```python
from build123d import *

# Parameters (mm, degrees)
BOX001_W          = 30
BOX001_H          = 70
BOX001_DEPTH      = 7.5
CYLINDER003_R     = 5
CYLINDER003_DEPTH = 40
CYLINDER002_R     = 17.5
CYLINDER002_DEPTH = 20


with BuildPart() as cube001:
    # Box001 → Box001 (new body)
    with BuildSketch(Plane(origin=(7, -20, 9), x_dir=(1, 0, 0), z_dir=(0, 0, 1))):
        with Locations((15, 35)):
            Rectangle(BOX001_W, BOX001_H)
    extrude(amount=BOX001_DEPTH)


with BuildPart() as cylinder003:
    # Cylinder003 → Cylinder003 (new body)
    with BuildSketch(Plane.XY.offset(-10)):
        Circle(CYLINDER003_R)
    extrude(amount=CYLINDER003_DEPTH)


with BuildPart() as mount_top:
    # Cylinder002 → Cylinder002 (new body)
    with BuildSketch(Plane.XY):
        Circle(CYLINDER002_R)
    extrude(amount=CYLINDER002_DEPTH)

    # Cut002: cut Cylinder003
    add(cylinder003.part, mode=Mode.SUBTRACT)

    # Cut003: cut Cube001
    add(cube001.part, mode=Mode.SUBTRACT)


solid = mount_top.part
```
Here's how the part is built. I have some questions about the finished solid (model axes, mm). A direction names the side the tool comes from. Coordinates: 2 decimals unless noted, no trailing zeros. Write each loop counter-clockwise with the first axis right and the second up, starting at its lowest first coordinate (ties: lowest second). Pieces come first, ordered by that corner, then holes. Notation, with made-up numbers: (10, 14.5) - (18, 14.5) arc R9 cw to (18, 23.5) - close; hole circle Ø4 at (-18.5, -7). An arc over 180 degrees is marked (long way). One line per item, written item: value.
1) Suppose I cut it at C-C on z = 3.25. Write out the boundary of the cut face in (x, y), and give its area (3 significant figures).
Model answer:
outline: circle Ø35 at (0, 0); hole circle Ø10 at (0, 0)
area: 884 mm²
2) Suppose I cut it at A-A on x = 0. Write out the boundary of the cut face in (y, z).
Model answer:
outline: (-17.5, 0) - (-5, 0) - (-5, 20) - (-17.5, 20) - close; (5, 0) - (17.5, 0) - (17.5, 20) - (5, 20) - close
3) I'm going to push flat-ended pins straight in: P1, Ø10, axis at x = -7.5, z = 7, coming from the -Y side; P2, Ø12, axis at x = 13.5, z = 8.5, coming from the -Y side; P3, Ø4, axis at x = 14, z = 12.5, coming from the +Y side; P4, Ø8, axis at y = -6.5, z = 5.5, coming from the +X side. Where does each tip first touch, or does it pass through?
Model answer:
P1: stops at y = -17.32
P2: stops at y = -15.81
P3: passes through
P4: stops at x = 17.32
4) I need wall thicknesses on line 1 along Y through (x, z) = (0, 11.75); line 2 along Z through (x, y) = (14.5, 6); line 3 along Y through (x, z) = (-4, 6). Which ranges of each line are inside material? Lowest first, please.
Model answer:
line 1: y = -17.5 to -5, 5 to 17.5
line 2: z = 0 to 9, 16.5 to 20
line 3: y = -17.04 to -3, 3 to 17.04
5) Suppose I cut it at B-B on y = 0. Write out the boundary of the cut face in (x, z).
Model answer:
outline: (-17.5, 0) - (-5, 0) - (-5, 20) - (-17.5, 20) - close; (5, 0) - (17.5, 0) - (17.5, 9) - (7, 9) - (7, 16.5) - (17.5, 16.5) - (17.5, 20) - (5, 20) - close
6) Suppose I cut it at D-D on y = -6.5. Write out the boundary of the cut face in (x, z).
Model answer:
outline: (-16.25, 0) - (16.25, 0) - (16.25, 9) - (7, 9) - (7, 16.5) - (16.25, 16.5) - (16.25, 20) - (-16.25, 20) - close
7) On a 3-axis mill with a long thin cutter (end or side, diameter ignored), from which of +Z, -Z, +X, -X, +Y, -Y can I reach the whole of each face in a straight line? I mean faces 5 (the flat face through (4, -4, 20)), 6 (the flat face through (11, 0, 9)). Say none if no direction works.
Model answer:
face 5: +Z, +X, -X, +Y, -Y
face 6: +X, +Y, -Y
8) We'd pull the mould along X, two halves only. Please class faces 1 (the flat face through (7, 0, 13)), 2 (the flat face through (4, -4, 0)), 3 (the cylindrical face through (-17.483, 0.769, 9.86)), 4 (the cylindrical face through (-1.08, -4.88, 9.86)): pulls with the +X half, pulls with the -X half, needs draft (parallel to the pull), parting line crosses it, or undercut.
Model answer:
face 1: pulls with the +X half
face 2: needs draft
face 3: parting line crosses it
face 4: undercut
